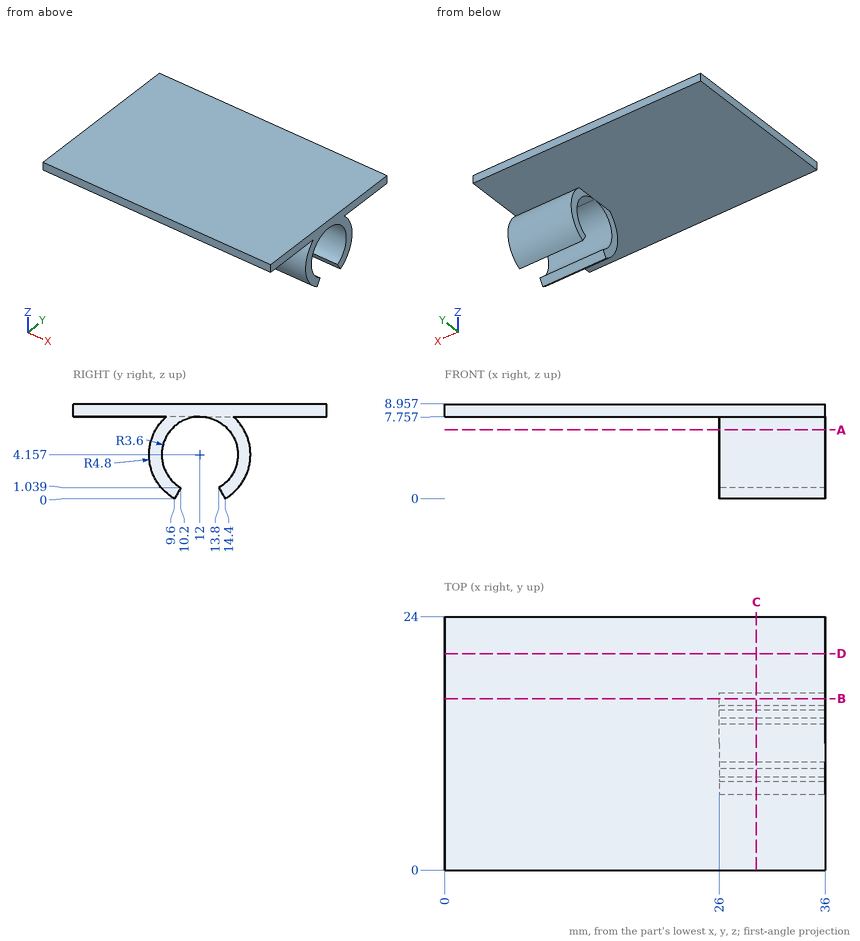
Answer from the drawing. Dimensions are ordinates in mm from the lowest x, y and z of the part. Give positions to 0.01 mm unless a question says otherwise; leave off trailing zeros. Write each loop counter-clockwise with the first axis right and the second up, starting at its lowest first coordinate (ties: lowest second). Pieces come first, ordered by that corner, then holes. Notation, with made-up numbers: (57.5, 40) -> (102.5, 40) arc R24 cw to (102.5, 75) -> close; hole circle Ø7 at (37, -1). An arc over 180 degrees is marked (long way). One line per question, with ' | ' between items. Start each with the question number.
1. Section D-D (y = 20.5) is taken. Determine the outline of the cut face in (x, z).
2. Section A-A (z = 6.5) is taken. Determine the outline of the cut face in (x, y).
3. Section B-B (y = 16.25) is taken. Determine the outline of the cut face in (x, z).
4. Find the intervals of material crossed by probe 1 along Z at (x, y) = (21, 19.5); probe 2 along X at (y, z) = (15.5, 6.5); probe 3 along Y at (x, z) = (28, 2), in increasing order.
5. Given pin 1 Ø2 at (x, z) = (31.5, 6.5) entering from -Y; pin 2 Ø1 at (x, z) = (15, 7.5) entering from -Y, each flat-ended and moving along its own axis, determine where each tip first touches the part or whether it passes through.
6. Section C-C (x = 29.5) is taken. Determine the outline of the cut face in (y, z) (1 decimal).
Response values:
1) outline: (0, 7.76) -> (36, 7.76) -> (36, 8.96) -> (0, 8.96) -> close
2) outline: (26, 7.81) -> (36, 7.81) -> (36, 9.27) -> (26, 9.27) -> close; (26, 14.73) -> (36, 14.73) -> (36, 16.19) -> (26, 16.19) -> close
3) outline: (0, 7.76) -> (36, 7.76) -> (36, 8.96) -> (0, 8.96) -> close; (26, 1.93) -> (36, 1.93) -> (36, 6.39) -> (26, 6.39) -> close
4) probe 1: 7.76 to 8.96 | probe 2: 26 to 36 | probe 3: 7.71 to 9.12, 14.88 to 16.29
5) pin 1: y = 7.39 | pin 2: y = 0
6) outline: (0, 7.8) -> (8.8, 7.8) arc R4.8 ccw to (9.6, 0) -> (10.2, 1) arc R3.6 cw (long way) to (13.8, 1) -> (14.4, 0) arc R4.8 ccw to (15.2, 7.8) -> (24, 7.8) -> (24, 9) -> (0, 9) -> close
